```python
from build123d import *

# Parameters (mm, degrees)
F1_DEPTH = 38.1
F2_R     = 6.35
F3_W     = 38.1
F3_H     = 101.6
F4_DEPTH = 38.1


with BuildPart() as f1:
    # F0 (on Right) → F1 (new body)
    with BuildSketch(Plane.YZ):
        with BuildLine():
            Line((-279.4, 0), (0, 0))
            Line((0, 0), (279.4, 0))
            ThreePointArc((279.4, 0), (256.466555, 72.795275), (195.948786, 119.300056))
            ThreePointArc((195.948786, 119.300056), (60.252824, 242.073318), (48.461383, 424.686653))
            Line((48.461383, 424.686653), (144.617616, 713.921884))
            ThreePointArc((144.617616, 713.921884), (150.441824, 737.648045), (152.4, 762))
            Line((152.4, 762), (76.2, 762))
            Line((76.2, 762), (0, 762))
            Line((0, 762), (-76.2, 762))
            Line((-76.2, 762), (-152.4, 762))
            ThreePointArc((-152.4, 762), (-150.441824, 737.648045), (-144.617616, 713.921884))
            Line((-144.617616, 713.921884), (-48.461383, 424.686653))
            ThreePointArc((-48.461383, 424.686653), (-60.252824, 242.073318), (-195.948786, 119.300056))
            ThreePointArc((-195.948786, 119.300056), (-256.466555, 72.795275), (-279.4, 0))
        make_face()
        Polygon((-76.2, 800.1), (-76.2, 762), (0, 762), (76.2, 762), (76.2, 800.1), align=None)
    extrude(amount=F1_DEPTH)

    # F2
    f2_edges = [f1.edges().sort_by_distance(p)[0] for p in [
        (38.1, -60.252824, 242.073318),
        (0, 60.252824, 242.073318),
        (38.1, 60.252824, 242.073318),
        (0, -96.539499, 569.304268),
    ]]
    fillet(f2_edges, radius=F2_R)

    # F3 (on face) → F4 (cut, through all)
    with BuildSketch(Plane(origin=(0, 0, 0), x_dir=(0, -1, 0), z_dir=(-1, 0, 0))):
        with Locations((0, 152.4)):
            Rectangle(F3_W, F3_H)
    extrude(amount=-F4_DEPTH, mode=Mode.SUBTRACT)


solid = f1.part
```
Read the model definition and answer for the solid it produces. Units are mm, in the model's axes. A direction names the side the tool comes from. Coordinates: 2 decimals unless noted, no trailing zeros. Loops run counter-clockwise (first coordinate to the right, second up) from the corner with the lowest first, then second, coordinate; pieces in that order, holes last. Notation, with made-up numbers: (-21, 63) -> (-9, 63) arc R12 cw to (-9, 81) -> close; hole circle Ø7 at (-24, 6). An arc over 180 degrees is marked (long way). Return JSON: item names as keys, results as strings.
Item 1: Flat-ended cylindrical pins translate along their axes: P1, Ø1, axis at x = 27.5, y = -151.5, coming from the +Z side; P2, Ø11.5, axis at x = 28.5, z = 146.5, coming from the -Y side; P3, Ø11.5, axis at x = 17.5, z = 774, coming from the -Y side. Find the tip coordinate at first contact, or state that the pin passes through.
Answers:
{"P1": "stops at z = 762", "P2": "stops at y = -151.68", "P3": "stops at y = -76.2"}
Item 2: For a pull along Y with two mould halves and no side action, classify faces 5 (the flat face through (19, -114, 762)), 6 (the cylindrical face through (18.872, -59.123, 244.445)), 7 (the cylindrical face through (18.87, 61.41, 239.71)), 8 (the flat face through (19, 0, 203.2)) as +Y half, -Y half, draft (parallel to the pull), parting line (faces both ways), or undercut.
Answers:
{"face 5": "draft", "face 6": "-Y half", "face 7": "+Y half", "face 8": "undercut"}
Item 3: For faces 1 (the flat face through (19, 19.05, 152)), 2 (the flat face through (18.872, -97.213, 571.329)), 3 (the flat face through (19, -76.2, 781)), 4 (the cylindrical face through (1.91, 95.494, 571.9)), determine the directions among +Z, -Z, +X, -X, +Y, -Y from which every point of the face is accessible in a straight line to the end or side of a thin tool.
Answers:
{"face 1": "+X, -X", "face 2": "+X, -X, -Y", "face 3": "+Z, +X, -X, -Y", "face 4": "-X, +Y"}
Item 4: Find section A-A (x = 13.5). Determine the outline of the cut face in (y, z).
Answers:
{"outline": "(-279.4, 0) -> (279.4, 0) arc R127 ccw to (195.95, 119.3) arc R243.37 cw to (48.46, 424.69) -> (144.62, 713.92) arc R152.4 ccw to (152.4, 762) -> (76.2, 762) -> (76.2, 800.1) -> (-76.2, 800.1) -> (-76.2, 762) -> (-152.4, 762) arc R152.4 ccw to (-144.62, 713.92) -> (-48.46, 424.69) arc R243.37 cw to (-195.95, 119.3) arc R127 ccw to start; hole (-19.05, 101.6) -> (19.05, 101.6) -> (19.05, 203.2) -> (-19.05, 203.2) -> close"}
Item 5: Find the intervals of material crossed by probe 1 along Z at (x, y) = (24, 10.5); probe 2 along Y at (x, z) = (26, 293); probe 3 along Y at (x, z) = (9.5, 764), in increasing order.
Answers:
{"probe 1": "z = 0 to 101.6, 203.2 to 800.1", "probe 2": "y = -42.31 to 42.31", "probe 3": "y = -76.2 to 76.2"}
